Source: CAD feature listing. Evaluate the final solid. Frame: model axes, mm. Round coordinates to 2 decimals unless told otherwise and drop trailing zeros. Loops run counter-clockwise (first coordinate to the right, second up) from the corner with the lowest first, then second, coordinate; pieces in that order, holes last. Notation, with made-up numbers: M 56.25,46 L 108.25,46 A23 ccw 108.25,54 Z; hole C 50,49 d6. An arc over 180 degrees is marked long. Write each question's results on one line, items separated by ' | '. Start each with the question number.
1. Section D-D on z = -1.1. Give the number of separate pieces and of enclosed holes in the cut face, and give its area (3 significant figures).
2. Ray query, line 1 (Y direction, x = 0, z = 0.1); line 2 (X direction, y = 2, z = -1.35); line 3 (X direction, y = -0.5, z = 1.5). Return the intervals inside material, ascending.
3. Draft query along X for faces 1 (the flat face through (0, 8, -1.75)), 2 (the cylindrical face through (-4.44, 33.81, 0.02)), 3 (the cylindrical face through (-13.56, 0.1, 0.02)). Return one class per face: released by +X, released by -X, zero draft, split by the parting line, or undercut.
4. Section C-C on x = 24.75. Output: boundary loops of the cut face in (y, z).
5. Section A-A on x = 0. Output: boundary loops of the cut face in (y, z), and give its area (3 significant figures).
6. Contact query for flat-ended pins moving along their axis: pin 1 Ø3 at (x, y) = (-1, 24) entering from +Z; pin 2 Ø1 at (y, z) = (24, -1) entering from -X; pin 3 Ø1 at (x, z) = (17.5, 1) entering from +Y; pin 4 Ø2 at (y, z) = (25.5, -0.5) entering from -X. Output: stop coordinate, or through.
from build123d import *

# Parameters (mm, degrees)
SKETCH1_R           = 34.1
BOSS_EXTRUDE1_DEPTH = 1.75
SKETCH3_R           = 2.25
CUT_EXTRUDE2_DEPTH  = 49.351525312
SKETCH2_R           = 7.25
CUT_EXTRUDE1_DEPTH  = 49.351525312


with BuildPart() as part:
    # Sketch1 → Boss-Extrude1 (new, symmetric)
    with BuildSketch(Plane.XY):
        Circle(SKETCH1_R)
    extrude(amount=BOSS_EXTRUDE1_DEPTH, both=True)

    # Sketch3 → Cut-Extrude2 (cut, through all)
    with BuildSketch(Plane.XY.offset(1.75)):
        with Locations((0, 24.75)):
            Circle(SKETCH3_R)
        with Locations((0, 11.3137085)):
            Circle(SKETCH3_R)
        with Locations((24.75, 0)):
            Circle(SKETCH3_R)
        with Locations((11.3137085, 0)):
            Circle(SKETCH3_R)
        with Locations((0, -24.75)):
            Circle(SKETCH3_R)
        with Locations((0, -11.3137085)):
            Circle(SKETCH3_R)
        with Locations((-24.75, 0)):
            Circle(SKETCH3_R)
        with Locations((-11.3137085, 0)):
            Circle(SKETCH3_R)
    extrude(amount=-CUT_EXTRUDE2_DEPTH, mode=Mode.SUBTRACT)

    # Sketch2 → Cut-Extrude1 (cut, through all)
    with BuildSketch(Plane.XY.offset(1.75)):
        Circle(SKETCH2_R)
    extrude(amount=-CUT_EXTRUDE1_DEPTH, mode=Mode.SUBTRACT)


solid = part.part
Taken from the geometry:
1) separate pieces: 1 | enclosed holes: 9 | area: 3,360 mm^2
2) line 1: -34.1 to -27, -22.5 to -13.56, -9.06 to -7.25, 7.25 to 9.06, 13.56 to 22.5, 27 to 34.1 | line 2: -34.04 to -25.78, -23.72 to -12.34, -10.28 to -6.97, 6.97 to 10.28, 12.34 to 23.72, 25.78 to 34.04 | line 3: -34.1 to -26.94, -22.56 to -13.51, -9.12 to -7.23, 7.23 to 9.12, 13.51 to 22.56, 26.94 to 34.1
3) face 1: zero draft | face 2: split by the parting line | face 3: undercut
4) outline: M -23.46,-1.75 L -2.25,-1.75 L -2.25,1.75 L -23.46,1.75 Z; M 2.25,-1.75 L 23.46,-1.75 L 23.46,1.75 L 2.25,1.75 Z
5) outline: M -34.1,-1.75 L -27,-1.75 L -27,1.75 L -34.1,1.75 Z; M -22.5,-1.75 L -13.56,-1.75 L -13.56,1.75 L -22.5,1.75 Z; M -9.06,-1.75 L -7.25,-1.75 L -7.25,1.75 L -9.06,1.75 Z; M 7.25,-1.75 L 9.06,-1.75 L 9.06,1.75 L 7.25,1.75 Z; M 13.56,-1.75 L 22.5,-1.75 L 22.5,1.75 L 13.56,1.75 Z; M 27,-1.75 L 34.1,-1.75 L 34.1,1.75 L 27,1.75 Z | area: 125 mm^2
6) pin 1: z = 1.75 | pin 2: x = -24.71 | pin 3: y = 29.56 | pin 4: x = -23.72
